```python
from build123d import *

# Parameters (mm, degrees)
SKETCH5_R          = 1.25
CUT_EXTRUDE1_DEPTH = 22
SKETCH6_R          = 7
CUT_EXTRUDE2_DEPTH = 15


with BuildPart() as part:
    # Surface-Knit1: read off the stored shape, not the designer's step
    # Surface-Knit1: loft between two sections, ruled curve by curve
    surface_knit1_from = [
        Edge.make_bspline([(2.083333333, 65, 0), (0.646232747, 64.800559216, 0), (-0.826702854, 64.515993467, 0), (-3.818616425, 63.749425521, 0), (-5.337603105, 63.267310443, 0), (-8.386455572, 62.082263598, 0), (-9.916283922, 61.37920281, 0), (-12.942411074, 59.736543691, 0), (-14.438613707, 58.796821883, 0), (-17.345798661, 56.676662259, 0), (-18.756625413, 55.496137115, 0), (-21.437875212, 52.905022069, 0), (-22.708100878, 51.494412766, 0), (-25.054855252, 48.47033026, 0), (-26.131181002, 46.856926203, 0), (-28.044894258, 43.470320821, 0), (-28.882119317, 41.697275034, 0), (-30.286104482, 38.046913607, 0), (-30.852782543, 36.169811281, 0), (-31.701669093, 32.373657167, 0), (-31.983893935, 30.454829684, 0), (-32.268420202, 26.637582521, 0), (-32.270825943, 24.73935017, 0), (-32.016934112, 21.019334498, 0), (-31.760796053, 19.197669041, 0), (-31.023611092, 15.67582868, 0), (-30.542738185, 13.975693203, 0), (-29.397291667, 10.728582673, 0), (-28.732872183, 9.18158041, 0), (-27.26390999, 6.258912542, 0), (-26.459481527, 4.883176255, 0), (-24.752359253, 2.309286831, 0), (-23.849734618, 1.111044068, 0), (-22.916666667, 0, 0)], [0, 0, 0, 0, 0.0625, 0.0625, 0.125, 0.125, 0.1875, 0.1875, 0.25, 0.25, 0.3125, 0.3125, 0.375, 0.375, 0.4375, 0.4375, 0.5, 0.5, 0.5625, 0.5625, 0.625, 0.625, 0.6875, 0.6875, 0.75, 0.75, 0.8125, 0.8125, 0.875, 0.875, 0.9375, 0.9375, 1, 1, 1, 1], 3),
        Edge.make_bspline([(27.083333333, 0, 0), (28.016401284, 1.111044068, 0), (28.91902592, 2.309286831, 0), (30.626148194, 4.883176255, 0), (31.430576657, 6.258912542, 0), (32.89953885, 9.18158041, 0), (33.563958334, 10.728582673, 0), (34.709404851, 13.975693203, 0), (35.190277759, 15.67582868, 0), (35.92746272, 19.197669041, 0), (36.183600779, 21.019334498, 0), (36.437492609, 24.73935017, 0), (36.435086869, 26.637582521, 0), (36.150560602, 30.454829684, 0), (35.868335759, 32.373657167, 0), (35.019449209, 36.169811281, 0), (34.452771148, 38.046913607, 0), (33.048785984, 41.697275034, 0), (32.211560925, 43.470320821, 0), (30.297847668, 46.856926203, 0), (29.221521919, 48.47033026, 0), (26.874767544, 51.494412766, 0), (25.604541879, 52.905022069, 0), (22.92329208, 55.496137115, 0), (21.512465328, 56.676662259, 0), (18.605280373, 58.796821883, 0), (17.10907774, 59.736543691, 0), (14.082950589, 61.37920281, 0), (12.553122239, 62.082263598, 0), (9.504269772, 63.267310443, 0), (7.985283092, 63.749425521, 0), (4.993369521, 64.515993467, 0), (3.52043392, 64.800559216, 0), (2.083333333, 65, 0)], [0, 0, 0, 0, 0.0625, 0.0625, 0.125, 0.125, 0.1875, 0.1875, 0.25, 0.25, 0.3125, 0.3125, 0.375, 0.375, 0.4375, 0.4375, 0.5, 0.5, 0.5625, 0.5625, 0.625, 0.625, 0.6875, 0.6875, 0.75, 0.75, 0.8125, 0.8125, 0.875, 0.875, 0.9375, 0.9375, 1, 1, 1, 1], 3),
        Edge.make_line((27.083333333, 0, 0), (-22.916666667, 0, 0)),
    ]
    surface_knit1_to = [
        Edge.make_bspline([(2.083333333, 65, 20), (0.647068043, 64.800424513, 20), (-0.824969306, 64.515786234, 20), (-3.814978177, 63.749245223, 20), (-5.332958295, 63.267229827, 20), (-8.379725343, 62.08260226, 20), (-9.908474817, 61.379861368, 20), (-12.932428528, 59.73810206, 20), (-14.427536732, 58.798960501, 20), (-17.332592911, 56.680243894, 20), (-18.742385636, 55.500581799, 20), (-21.421715644, 52.911470639, 20), (-22.691056015, 51.502002286, 20), (-25.036276618, 48.480441163, 20), (-26.111954405, 46.8684174, 20), (-28.024682221, 43.48474031, 20), (-28.861570209, 41.713242126, 20), (-30.265236079, 38.066046457, 20), (-30.831932078, 36.190561729, 20), (-31.681215411, 32.397605605, 20), (-31.963818965, 30.480357956, 20), (-32.24943077, 26.666132321, 20), (-32.252542967, 24.76934126, 20), (-32.000328363, 21.051990902, 20), (-31.745160599, 19.231549308, 20), (-31.010098955, 15.711890824, 20), (-30.530378628, 14.01271343, 20), (-29.387334902, 10.767236468, 20), (-28.724165314, 9.220909913, 20), (-27.257723578, 6.29932121, 20), (-26.454565517, 4.923988664, 20), (-24.749943011, 2.350663913, 20), (-23.848547718, 1.152582349, 20), (-22.916666667, 0.041598071, 20)], [0, 0, 0, 0, 0.0625, 0.0625, 0.125, 0.125, 0.1875, 0.1875, 0.25, 0.25, 0.3125, 0.3125, 0.375, 0.375, 0.4375, 0.4375, 0.5, 0.5, 0.5625, 0.5625, 0.625, 0.625, 0.6875, 0.6875, 0.75, 0.75, 0.8125, 0.8125, 0.875, 0.875, 0.9375, 0.9375, 1, 1, 1, 1], 3),
        Edge.make_bspline([(27.083333333, 0.041598071, 20), (28.013324474, 1.15416485, 20), (28.912650953, 2.353624766, 20), (30.612882601, 4.929167074, 20), (31.413718634, 6.305337934, 20), (32.875425295, 9.227959299, 20), (33.536182318, 10.774479235, 20), (34.674523423, 14.019650076, 20), (35.151954723, 15.718327197, 20), (35.882803171, 19.236326493, 20), (36.136048243, 21.05560894, 20), (36.385015288, 24.770116129, 20), (36.380579809, 26.665223747, 20), (36.093095417, 30.475786604, 20), (35.809943747, 32.391056326, 20), (34.960413899, 36.18005484, 20), (34.394019828, 38.053561803, 20), (32.991758511, 41.697107973, 20), (32.155972434, 43.466936274, 20), (30.246080794, 46.847842163, 20), (29.172135744, 48.458765813, 20), (26.830760169, 51.478864648, 20), (25.563530264, 52.887971076, 20), (22.888516003, 55.477149894, 20), (21.480926996, 56.657240939, 20), (18.58010928, 58.777551077, 20), (17.087034883, 59.717856056, 20), (14.066775655, 61.362540967, 20), (12.539686611, 62.06704278, 20), (9.495740577, 63.255611058, 20), (7.978921334, 63.739805204, 20), (4.990683697, 64.510935324, 20), (3.51925729, 64.797983291, 20), (2.083333333, 65, 20)], [0, 0, 0, 0, 0.0625, 0.0625, 0.125, 0.125, 0.1875, 0.1875, 0.25, 0.25, 0.3125, 0.3125, 0.375, 0.375, 0.4375, 0.4375, 0.5, 0.5, 0.5625, 0.5625, 0.625, 0.625, 0.6875, 0.6875, 0.75, 0.75, 0.8125, 0.8125, 0.875, 0.875, 0.9375, 0.9375, 1, 1, 1, 1], 3),
        Edge.make_line((27.083333333, 0.041598071, 20), (-22.916666667, 0.041598071, 20)),
    ]
    surface_knit1 = Solid(Shell([*[Face.make_surface_from_curves(surface_knit1_from[k], surface_knit1_to[k]) for k in range(3)], Face(Wire(surface_knit1_from)), Face(Wire(surface_knit1_to))]))
    add(surface_knit1)

    # Sketch5 → Cut-Extrude1 (cut)
    with BuildSketch(Plane.XY.offset(20)):
        with Locations((-2.616666667, 13.268765789)):
            Circle(SKETCH5_R)
        with Locations((-2.916666667, 60.888765789)):
            Circle(SKETCH5_R)
        with Locations(Location((6.783333333, 13.268765789, 0), (0, 0, 180))):
            Circle(SKETCH5_R)
        with Locations(Location((7.083333333, 60.888765789, 0), (0, 0, 180))):
            Circle(SKETCH5_R)
        Polygon((12.583333333, 16.078765789), (-8.416666667, 16.078765789), (-8.416666667, 58.078765789), (-0.916666667, 58.078765789), (-0.916666667, 65.078765789), (5.083333333, 65.078765789), (5.083333333, 58.078765789), (12.583333333, 58.078765789), align=None)
    extrude(amount=-CUT_EXTRUDE1_DEPTH, mode=Mode.SUBTRACT)

    # Sketch6 → Cut-Extrude2 (cut)
    with BuildSketch(Plane(origin=(0, 0, 0), x_dir=(1, 0, 0), z_dir=(0, 1, 0))):
        with Locations(Location((-14.916666667, -10, 0), (0, 0, 90))):
            Circle(SKETCH6_R)
        with Locations(Location((19.083333333, -10, 0), (0, 0, 90))):
            Circle(SKETCH6_R)
    extrude(amount=CUT_EXTRUDE2_DEPTH, mode=Mode.SUBTRACT)


solid = part.part
```
Read the model definition and answer for the solid it produces. Units are mm, in the model's axes. A direction names the side the tool comes from. Give positions to 0.01 mm unless a question says otherwise; leave off trailing zeros.
Item 1: For faces 3 (the flat face through (-15, 15, 10)), 4 (the flat face through (2, 16.079, 10)), 5 (the flat face through (2, 11, 0)), 6 (the flat face through (-0.917, 61, 10)), determine the directions among +Z, -Z, +X, -X, +Y, -Y from which every point of the face is accessible in a straight line to the end or side of a thin tool.
Item 2: The part is cut by section A-A (z = 6.25). Give the number of separate pieces and of enclosed holes in the cut face, and give its area (3 significant figures).
Item 3: Each of these flat-tipped pins is pushed along its axis until it touches: pin 1 Ø10 at (x, z) = (3, 6.5) entering from +Y; pin 2 Ø5 at (x, z) = (-14.5, 8) entering from +Y; pin 3 Ø6 at (y, z) = (41.5, 5.5) entering from -X; pin 4 Ø11 at (x, z) = (-16.5, 9.5) entering from -Y. Where does it stop, or does it pass through?
Item 4: The mould has two halves that part along X. Classify faces 1 (the cylindrical face through (-3.08, 62.13, 10.14)), 2 (the flat face through (2, 11, 20)): released by +X, released by -X, zero draft, split by the parting line, or undercut.
Item 5: Find the intervals of material crossed by line 1 along X through (y, z) = (13, 11.5); line 2 along X through (y, z) = (8, 10); line 3 along Y through (x, z) = (11.5, 16.75), in increasing order.
Taken from the geometry:
1. face 3: -Y
1. face 4: +Z, -Z
1. face 5: -Z, +X, -X, +Y, -Y
1. face 6: +Z, -Z, +Y
2. separate pieces: 1
2. enclosed holes: 4
2. area: 2,360 mm2
3. pin 1: stops at y = 64.47
3. pin 2: stops at y = 60.24
3. pin 3: stops at x = -30.08
3. pin 4: stops at y = 0.01
4. face 1: undercut
4. face 2: zero draft
5. line 1: x = -30.18 to -21.75, -8.08 to -3.84, -1.4 to 5.56, 8 to 12.25, 25.92 to 34.33
5. line 2: x = -28.12 to -21.92, -7.92 to 12.08, 26.08 to 32.28
5. line 3: y = 0.03 to 16.08, 58.08 to 62.47
